Can you work these out from the model? Positions are in its coordinate system, mm. Face numbers are marked on the shaded views. A direction names the side the tool comes from. Give positions to 0.01 mm unless a question says otherwise; leave off trailing zeros. Order: outer loops, then holes, each group sorted by start corner. A loop starts at its lowest first (then second) coordinate and runs counter-clockwise, first axis right, second up. Notation, with made-up numbers: M 77,60.25 L 83,60.25 A11 cw 83,74.25 Z; hole C 49,59.5 d1. An arc over 180 degrees is marked long. Write each question's results on one line, items separated by ' | '.
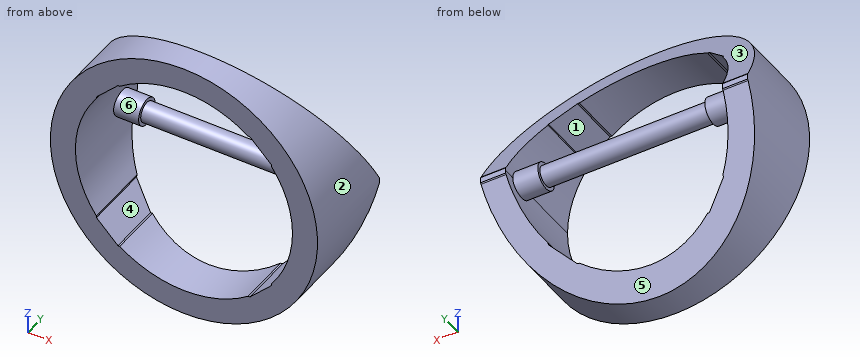
from build123d import *

# Parameters (mm, degrees)
ESQUISSE2_R             = 400
BOSS_EXTRU_1_DEPTH      = 300
ENL_V_MAT_EXTRU_1_DEPTH = 575
ENL_V_START             = 705
ENL_V_MAT_EXTRU_2_DEPTH = 705
ESQUISSE9_R             = 40
BOSS_EXTRU_10_DEPTH     = 350
BOSS_EXTRU_11_START     = -350
ESQUISSE9_4_R           = 40
BOSS_EXTRU_11_DEPTH     = 350
ENL_V_START_2           = -250
ESQUISSE10_R            = 40
ESQUISSE10_R_2          = 30
ENL_V_MAT_EXTRU_3_DEPTH = 250
ESQUISSE10_2_R          = 40
ESQUISSE10_2_R_2        = 30
ENL_V_MAT_EXTRU_4_DEPTH = 250


with BuildPart() as part:
    # Esquisse2 → Boss.-Extru.1 (new body)
    with BuildSketch(Plane(origin=(0, 0, 0), x_dir=(1, 0, 0), z_dir=(0, 1, 0))):
        with Locations(Location((0, 0, 0), (0, 0, 270))):
            Circle(ESQUISSE2_R)
        with BuildLine():
            Line((-262.027957955, 192.26634976), (-262.027957955, 197.591449816))
            Line((-262.027957955, 197.591449816), (-229.809703961, 229.80970381))
            Line((-229.809703961, 229.80970381), (-197.591449816, 262.027957955))
            Line((-197.591449816, 262.027957955), (-192.26634976, 262.027957955))
            ThreePointArc((-192.26634976, 262.027957955), (0, 325), (192.26634976, 262.027957955))
            Line((192.26634976, 262.027957955), (197.591449816, 262.027957955))
            Line((197.591449816, 262.027957955), (229.809703566, 229.809704205))
            Line((229.809703566, 229.809704205), (262.027957955, 197.591449816))
            Line((262.027957955, 197.591449816), (262.027957955, 192.26634976))
            ThreePointArc((262.027957955, 192.26634976), (308.856023363, 101.158078433), (325, 0))
            ThreePointArc((325, 0), (308.856023363, -101.158078433), (262.027957955, -192.26634976))
            Line((262.027957955, -192.26634976), (262.027957955, -197.591449816))
            Line((262.027957955, -197.591449816), (229.809704204, -229.809703567))
            Line((229.809704204, -229.809703567), (197.591449816, -262.027957955))
            Line((197.591449816, -262.027957955), (192.26634976, -262.027957955))
            ThreePointArc((192.26634976, -262.027957955), (0, -325), (-192.26634976, -262.027957955))
            Line((-192.26634976, -262.027957955), (-197.591449816, -262.027957955))
            Line((-197.591449816, -262.027957955), (-229.809704607, -229.809703164))
            Line((-229.809704607, -229.809703164), (-262.027957955, -197.591449816))
            Line((-262.027957955, -197.591449816), (-262.027957955, -192.26634976))
            ThreePointArc((-262.027957955, -192.26634976), (-325, 0), (-262.027957955, 192.26634976))
        make_face(mode=Mode.SUBTRACT)
    extrude(amount=BOSS_EXTRU_1_DEPTH)

    # Esquisse3 → Enl_v. mat.-Extru.1 (cut)
    with BuildSketch(Plane(origin=(0, 0, 0), x_dir=(0, 0, -1), z_dir=(1, 0, 0))):
        with BuildLine():
            ThreePointArc((-11.82699013, 297.660323463), (-8.312403851, 300.008694936), (-4.166666667, 300.833333333))
            Line((-4.166666667, 300.833333333), (-400, 300.833333333))
            Line((-400, 300.833333333), (-400, 80.833333333))
            Line((-400, 80.833333333), (-11.82699013, 297.660323463))
        make_face()
        with BuildLine():
            Line((400, 300.833333333), (4.166666667, 300.833333333))
            ThreePointArc((4.166666667, 300.833333333), (8.312403851, 300.008694936), (11.82699013, 297.660323463))
            Line((11.82699013, 297.660323463), (400, 80.833333333))
            Line((400, 80.833333333), (400, 300.833333333))
        make_face()
    extrude(amount=-ENL_V_MAT_EXTRU_1_DEPTH, mode=Mode.SUBTRACT)

    # Esquisse3_3 → Enl_v. mat.-Extru.2 (cut)
    with BuildSketch(Plane(origin=(0, 0, 0), x_dir=(0, 0, -1), z_dir=(1, 0, 0)).offset(ENL_V_START)):
        with BuildLine():
            ThreePointArc((-11.82699013, 297.660323463), (-8.312403851, 300.008694936), (-4.166666667, 300.833333333))
            Line((-4.166666667, 300.833333333), (-400, 300.833333333))
            Line((-400, 300.833333333), (-400, 80.833333333))
            Line((-400, 80.833333333), (-11.82699013, 297.660323463))
        make_face()
        with BuildLine():
            Line((400, 300.833333333), (4.166666667, 300.833333333))
            ThreePointArc((4.166666667, 300.833333333), (8.312403851, 300.008694936), (11.82699013, 297.660323463))
            Line((11.82699013, 297.660323463), (400, 80.833333333))
            Line((400, 80.833333333), (400, 300.833333333))
        make_face()
    extrude(amount=-ENL_V_MAT_EXTRU_2_DEPTH, mode=Mode.SUBTRACT)

    # Esquisse9 → Boss.-Extru.10 (add)
    with BuildSketch(Plane(origin=(0, 0, 0), x_dir=(0, 0, -1), z_dir=(1, 0, 0))):
        with Locations(Location((0, 225, 0), (0, 0, 180))):
            Circle(ESQUISSE9_R)
    extrude(amount=BOSS_EXTRU_10_DEPTH)

    # Esquisse9_4 → Boss.-Extru.11 (add)
    with BuildSketch(Plane(origin=(0, 0, 0), x_dir=(0, 0, -1), z_dir=(1, 0, 0)).offset(BOSS_EXTRU_11_START)):
        with Locations(Location((0, 225, 0), (0, 0, 180))):
            Circle(ESQUISSE9_4_R)
    extrude(amount=BOSS_EXTRU_11_DEPTH)

    # Esquisse10 → Enl_v. mat.-Extru.3 (cut)
    with BuildSketch(Plane(origin=(0, 0, 0), x_dir=(0, 0, -1), z_dir=(1, 0, 0)).offset(ENL_V_START_2)):
        with Locations((0, 225)):
            Circle(ESQUISSE10_R)
        with Locations((0, 225)):
            Circle(ESQUISSE10_R_2, mode=Mode.SUBTRACT)
    extrude(amount=ENL_V_MAT_EXTRU_3_DEPTH, mode=Mode.SUBTRACT)

    # Esquisse10_2 → Enl_v. mat.-Extru.4 (cut)
    with BuildSketch(Plane(origin=(0, 0, 0), x_dir=(0, 0, -1), z_dir=(1, 0, 0))):
        with Locations((0, 225)):
            Circle(ESQUISSE10_2_R)
        with Locations((0, 225)):
            Circle(ESQUISSE10_2_R_2, mode=Mode.SUBTRACT)
    extrude(amount=ENL_V_MAT_EXTRU_4_DEPTH, mode=Mode.SUBTRACT)


solid = part.part
(1) We'd pull the mould along X, two halves only. Please class the marked faces 1, 2 and 3: +X half, -X half, draft (parallel to the pull), parting line (faces both ways), or undercut.
Data:
face 1: undercut | face 2: parting line | face 3: draft
(2) Imagine slicing it at D-D, the plane y = 225. Write out the boundary of the cut face in (x, z), plus the area to 3 significant figures.
Data:
outline: M -373.98,-141.91 L -292.38,-141.91 A325 cw -322.53,-40 L -250,-40 L -250,-30 L 250,-30 L 250,-40 L 322.53,-40 A325 cw 292.38,-141.91 L 373.98,-141.91 A400 ccw 373.98,141.91 L 292.38,141.91 A325 cw 322.53,40 L 250,40 L 250,30 L -250,30 L -250,40 L -322.53,40 A325 cw -292.38,141.91 L -373.98,141.91 A400 ccw Z | area: 85,600 mm2
(3) For the marked faces 4, 5 and 6, which set-ups out of +Z, -Z, +X, -X, +Y, -Y let a thin tool reach every point of the face, with its end or its side?
Data:
face 4: +Y, -Y | face 5: -Z, +X, -X, +Y | face 6: none
(4) Imagine slicing it at C-C, the plane x = 135.5. Write out the boundary of the cut face in (y, z).
Data:
outline: M 0,-376.35 L 94.04,-376.35 L 139.26,-295.41 L 0,-295.41 Z; M 0,295.41 L 139.26,295.41 L 94.04,376.35 L 0,376.35 Z; C 225,0 d60
(5) Imagine slicing it at A-A, the plane z = 62. Write out the boundary of the cut face in (x, y), plus the area to 3 significant figures.
Data:
outline: M -395.17,0 L -319.03,0 L -319.03,269.63 L -395.17,269.63 Z; M 319.03,0 L 395.17,0 L 395.17,269.63 L 319.03,269.63 Z | area: 41,100 mm2
(6) I need wall thicknesses on L1, parallel to Z at x = -36.5, y = 54; L2, parallel to X at y = 234.5, z = 105; L3, parallel to X at y = 24, z = -71.5. Which ranges of each line are inside material? Lowest first, please. Write a range as from..to.
Data:
L1: z = -398.33..-322.94, 322.94..398.33 | L2: x = -385.97..-307.57, 307.57..385.97 | L3: x = -393.56..-317.04, 317.04..393.56
(7) Will these pins go through, and if not, where does the flat tip stop? P1, Ø1.6, axis at y = 139, z = 196, coming from the +X side; P2, Ø6, axis at x = 194.5, y = 66, coming from the -Z side; P3, Ø1.6, axis at x = -195, y = 81, coming from the +Z side.
Data:
P1: stops at x = 349.14 | P2: stops at z = -351.18 | P3: stops at z = 349.69
(8) Imagine slicing it at B-B, the plane y = 36. Write out the boundary of the cut face in (x, z), plus the area to 3 significant figures.
Data:
outline: C 0,0 d800; hole M -262.03,-197.59 L -197.59,-262.03 L -192.27,-262.03 A325 ccw 192.27,-262.03 L 197.59,-262.03 L 262.03,-197.59 L 262.03,-192.27 A325 ccw 262.03,192.27 L 262.03,197.59 L 197.59,262.03 L 192.27,262.03 A325 ccw -192.27,262.03 L -197.59,262.03 L -262.03,197.59 L -262.03,192.27 A325 ccw -262.03,-192.27 Z | area: 170,000 mm2
